Can you work these out from the model? Positions are in its coordinate system, mm. Round coordinates to 2 decimals unless told otherwise and drop trailing zeros. Loops run counter-clockwise (first coordinate to the right, second up) from the corner with the lowest first, then second, coordinate; pieces in that order, holes last.
(1) I want a section at A-A on z = -130.5. Write out the boundary of the cut face in (x, y), plus the area to 3 significant figures.
(2) I want a section at C-C on x = 96. Write out the boundary of the cut face in (y, z), plus the area to 3 significant figures.
(3) Will these pins go through, and if not, where does the flat tip stop? pin 1 Ø1.4 at (y, z) = (1.5, -50) entering from -X; pin 2 Ø2.5 at (x, y) = (85.5, 3.5) entering from -Z; pin 3 Ø2.5 at (x, y) = (58.5, 2) entering from +Z.
(4) I want a section at D-D on x = 58.5. Write out the boundary of the cut face in (y, z), plus the area to 3 significant figures.
(5) I want a section at B-B on z = -107. Write out the boundary of the cut face in (x, y), plus the area to 3 significant figures.
(6) If I drill on line 1 along X through (y, z) = (4.4, -142); line 2 along X through (y, z) = (2.7, -106); line 3 along Z through (x, y) = (113, 0.4), over which ranges is the centre line in solid material (lowest first)?
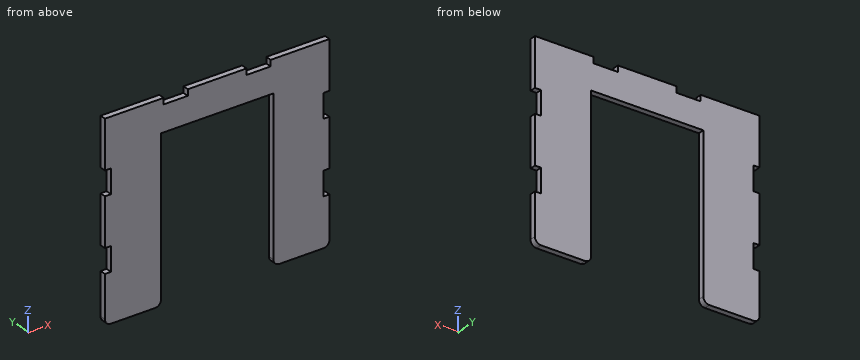
from build123d import *

# Parameters (mm, degrees)
SKETCH1_W             = 177.8
SKETCH1_H             = 152.4
BOSS_EXTRUDE1_DEPTH   = 4.826
SKETCH2_W             = 88.9
SKETCH2_H             = 127
CENTER_CUTOUT_DEPTH   = 235.22615199
SKETCH3_W             = 19.05
SKETCH3_H             = 4.826
BACK_EDGE_SLOTS_DEPTH = 235.22615199
SKETCH5_W             = 4.826
SKETCH5_H             = 19.05
SIDE_EDGE_SLOTS_DEPTH = 235.22615199
LEADING_EDGE_FILLET_R = 4.826


with BuildPart() as part:
    # Sketch1 → Boss-Extrude1 (new body)
    with BuildSketch(Plane(origin=(0, 0, 0), x_dir=(1, 0, 0), z_dir=(0, 1, 0))):
        with Locations((88.9, 76.2)):
            Rectangle(SKETCH1_W, SKETCH1_H)
    extrude(amount=BOSS_EXTRUDE1_DEPTH)

    # Sketch2 → Center Cutout (cut, through all)
    with BuildSketch(Plane(origin=(0, 4.826, 0), x_dir=(1, 0, 0), z_dir=(0, 1, 0))):
        with Locations((88.9, 88.9)):
            Rectangle(SKETCH2_W, SKETCH2_H)
    extrude(amount=-CENTER_CUTOUT_DEPTH, mode=Mode.SUBTRACT)

    # Sketch3 → Back Edge Slots (cut, through all)
    with BuildSketch(Plane(origin=(0, 4.826, 0), x_dir=(1, 0, 0), z_dir=(0, 1, 0))):
        with Locations((56.091666667, 2.413)):
            Rectangle(SKETCH3_W, SKETCH3_H)
        with Locations((121.708333333, 2.413)):
            Rectangle(SKETCH3_W, SKETCH3_H)
    extrude(amount=-BACK_EDGE_SLOTS_DEPTH, mode=Mode.SUBTRACT)

    # Sketch5 → Side Edge Slots (cut, through all)
    with BuildSketch(Plane(origin=(0, 4.826, 0), x_dir=(1, 0, 0), z_dir=(0, 1, 0))):
        with Locations((2.413, 104.775)):
            Rectangle(SKETCH5_W, SKETCH5_H)
        with Locations((2.413, 47.625)):
            Rectangle(SKETCH5_W, SKETCH5_H)
        with Locations((175.387, 104.775)):
            Rectangle(SKETCH5_W, SKETCH5_H)
        with Locations((175.387, 47.625)):
            Rectangle(SKETCH5_W, SKETCH5_H)
    extrude(amount=-SIDE_EDGE_SLOTS_DEPTH, mode=Mode.SUBTRACT)

    # Leading Edge Fillet
    leading_edge_fillet_edges = [part.edges().sort_by_distance(p)[0] for p in [
        (44.45, 2.413, -152.4),
        (133.35, 2.413, -152.4),
        (0, 2.413, -152.4),
        (177.8, 2.413, -152.4),
    ]]
    fillet(leading_edge_fillet_edges, radius=LEADING_EDGE_FILLET_R)


solid = part.part
Filled sheet:
1. outline: (0, 0) - (44.45, 0) - (44.45, 4.83) - (0, 4.83) - close; (133.35, 0) - (177.8, 0) - (177.8, 4.83) - (133.35, 4.83) - close
1. area: 429 mm2
2. outline: (0, -25.4) - (4.83, -25.4) - (4.83, 0) - (0, 0) - close
2. area: 123 mm2
3. pin 1: stops at x = 4.83
3. pin 2: stops at z = -25.4
3. pin 3: stops at z = -4.83
4. outline: (0, -25.4) - (4.83, -25.4) - (4.83, -4.83) - (0, -4.83) - close
4. area: 99.3 mm2
5. outline: (4.83, 0) - (44.45, 0) - (44.45, 4.83) - (4.83, 4.83) - close; (133.35, 0) - (172.97, 0) - (172.97, 4.83) - (133.35, 4.83) - close
5. area: 382 mm2
6. line 1: x = 0 to 44.45, 133.35 to 177.8
6. line 2: x = 4.83 to 44.45, 133.35 to 172.97
6. line 3: z = -25.4 to -4.83
